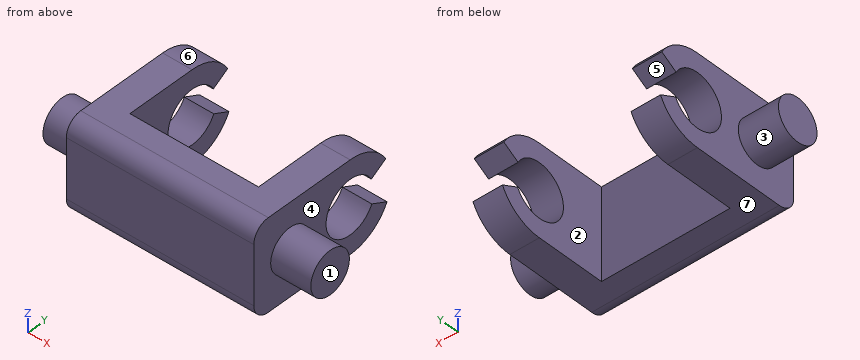
from build123d import *

# Parameters (mm, degrees)
SKETCH1_R               = 8
BOSS_EXTRUDE1_DEPTH     = 50
SKETCH2_R               = 10
BOSS_EXTRUDE2_DEPTH     = 35
CUT_EXTRUDE1_DEPTH      = 68.475921631
CUT_EXTRUDE1_DEPTH_BACK = 68.475921631
SKETCH3_W               = 48
SKETCH3_H               = 42.81
CUT_EXTRUDE2_REACH      = 98.322


with BuildPart() as part:
    # Sketch1 → Boss-Extrude1 (new, symmetric)
    with BuildSketch(Plane(origin=(0, 0, 0), x_dir=(0, 0, -1), z_dir=(1, 0, 0))):
        Circle(SKETCH1_R)
    extrude(amount=BOSS_EXTRUDE1_DEPTH, both=True)

    # Sketch2 → Boss-Extrude2 (add, symmetric)
    with BuildSketch(Plane(origin=(0, 0, 0), x_dir=(0, 0, -1), z_dir=(1, 0, 0))):
        with BuildLine():
            Line((-11, -15), (11, -15))
            ThreePointArc((11, -15), (15.242640687, -13.242640687), (17, -9))
            Line((17, -9), (17, 25))
            ThreePointArc((17, 25), (0, 42), (-17, 25))
            Line((-17, 25), (-17, -9))
            ThreePointArc((-17, -9), (-15.242640687, -13.242640687), (-11, -15))
        make_face()
        with Locations((0, 25)):
            Circle(SKETCH2_R, mode=Mode.SUBTRACT)
    extrude(amount=BOSS_EXTRUDE2_DEPTH, both=True)

    # Sketch3 → Cut-Extrude1 (cut, two sides: drawn at the far end of the back side and taken through both)
    with BuildSketch(Plane.XY.offset(-CUT_EXTRUDE1_DEPTH_BACK)):
        with Locations((0, 20.595)):
            Rectangle(SKETCH3_W, SKETCH3_H)
    extrude(amount=CUT_EXTRUDE1_DEPTH + CUT_EXTRUDE1_DEPTH_BACK, mode=Mode.SUBTRACT)

    # Cut-Extrude2: up to this face of the body (flat: up to its plane)
    cut_extrude2_end = Plane(part.part.faces().sort_by_distance((-35, 10.739149223, 0))[0])
    # Sketch4 → Cut-Extrude2 (cut, up to the picked face)
    with BuildSketch(Plane(origin=(35, 0, 0), x_dir=(0, 0, -1), z_dir=(1, 0, 0)), mode=Mode.PRIVATE) as cut_extrude2_sk1:
        with BuildLine():
            Line((-8.398206087, 39.78073525), (-4.706155375, 33.823383795))
            ThreePointArc((-4.706155375, 33.823383795), (-0.206218371, 34.997873473), (4.338321313, 34.009937191))
            Line((4.338321313, 34.009937191), (7.375146233, 40.316893224))
            ThreePointArc((7.375146233, 40.316893224), (-0.577519878, 41.990187485), (-8.398206087, 39.78073525))
        make_face()
    cut_extrude2_tool1 = split(extrude(cut_extrude2_sk1.sketch, amount=-CUT_EXTRUDE2_REACH, mode=Mode.PRIVATE), bisect_by=cut_extrude2_end, keep=Keep.BOTH, mode=Mode.PRIVATE)
    add(cut_extrude2_tool1.solids().sort_by(Axis((35, 38.290838, 0.393307), (-1, 0, 0)))[0], mode=Mode.SUBTRACT)


solid = part.part
Source: CAD feature listing. Evaluate the final solid. Frame: model axes, mm. Face numbers are marked on the shaded views. A direction names the side the tool comes from. Round coordinates to 2 decimals unless told otherwise and drop trailing zeros. Loops run counter-clockwise (first coordinate to the right, second up) from the corner with the lowest first, then second, coordinate; pieces in that order, holes last.
Q1. Ray query, line 1 (X direction, y = 29.5, z = -9); line 2 (X direction, y = 1, z = 1.5); line 3 (Z direction, x = 30.5, y = 25). Return the intervals inside material, ascending.
Q2. First-contact query: P1, Ø10, axis at y = 28, z = 2, coming from the +X side; P2, Ø1.5, axis at x = -38, z = -1.5, coming from the +Y side; P3, Ø2, axis at x = 16, z = -5.5, coming from the +Y side; P4, Ø5, axis at y = 32.5, z = -3.5, coming from the +X side. Flat tips, straight axial feed; report the tip coordinate or a pass-through.
Q3. Section A-A, the plane y = 11. Return loops of the section in (x, z), plus the area to 3 significant figures.
Q4. Section B-B, the plane z = 0. Return loops of the section in (x, y).
Q5. Section D-D, the plane x = -16. Return loops of the section in (y, z).
Q6. Section C-C, the plane y = 30. Return loops of the section in (x, z).
Q7. Mould query, pull axis Z, two halves, no side actions, for the marked faces 5, 6 and 7. Classes: pulls with the +Z half, pulls with the -Z half, needs draft (parallel to the pull), parting line crosses it, or undercut.
Q8. Access query for the marked faces 1, 2, 3 and 4. Directions: +Z, -Z, +X, -X, +Y, -Y. A direction counts if a zero-diameter tool reaches every point of the face in a straight line with its end or side. Return the directions, or none.
Solutions:
1. line 1: x = -35 to -24, 24 to 35
1. line 2: x = -50 to -24, 24 to 50
1. line 3: z = -17 to -10, 10 to 17
2. P1: passes through
2. P2: stops at y = 7.96
2. P3: stops at y = -0.81
2. P4: stops at x = 35
3. outline: (-35, -17) - (-24, -17) - (-24, 17) - (-35, 17) - close; (24, -17) - (35, -17) - (35, 17) - (24, 17) - close
3. area: 748 mm2
4. outline: (-50, -8) - (-35, -8) - (-35, -15) - (35, -15) - (35, -8) - (50, -8) - (50, 8) - (35, 8) - (35, 15) - (24, 15) - (24, -0.81) - (-24, -0.81) - (-24, 15) - (-35, 15) - (-35, 8) - (-50, 8) - close
5. outline: (-15, -11) arc R6 ccw to (-9, -17) - (-0.81, -17) - (-0.81, 17) - (-9, 17) arc R6 ccw to (-15, 11) - close
6. outline: (-35, -16.25) - (-24, -16.25) - (-24, -8.66) - (-35, -8.66) - close; (-35, 8.66) - (-24, 8.66) - (-24, 16.25) - (-35, 16.25) - close; (24, -16.25) - (35, -16.25) - (35, -8.66) - (24, -8.66) - close; (24, 8.66) - (35, 8.66) - (35, 16.25) - (24, 16.25) - close
7. face 5: undercut
7. face 6: pulls with the +Z half
7. face 7: pulls with the -Z half
8. face 1: +Z, -Z, +X, +Y, -Y
8. face 2: +Z, -Z, +Y
8. face 3: -X
8. face 4: +X
